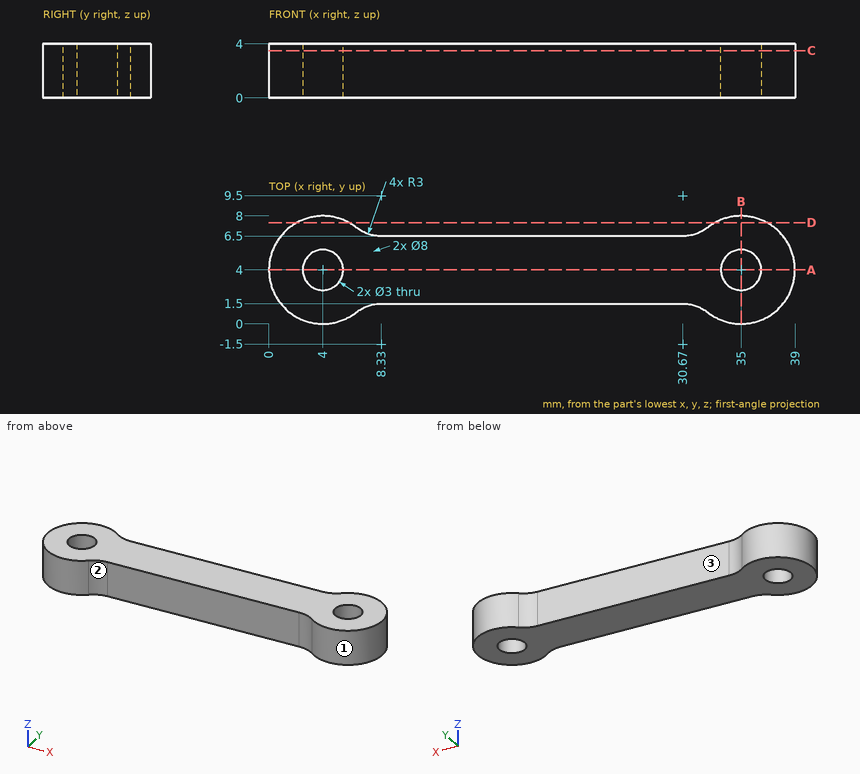
Check sheet for the drawn part. Datum: minimum x, y, z corner. Units: mm. A direction names the side the tool comes from. Round coordinates to 2 decimals unless told otherwise and drop trailing zeros. Loops run counter-clockwise (first coordinate to the right, second up) from the corner with the lowest first, then second, coordinate; pieces in that order, holes last. Notation, with made-up numbers: (-2.5, 43) - (15.5, 43) arc R32 ccw to (15.5, 82) - close; hole circle Ø11 at (17, 11.5). An arc over 180 degrees is marked (long way). Write each question's results on one line, items separated by ' | '. Start each with the question number.
Q1. Cross-section at B-B on x = 35. Enter the section's corners in (y, z), and give its area (3 significant figures).
Q2. Gauge pin test, flat ends, axial feed: P1, Ø1.5, axis at x = 21, z = 1.5, coming from the -Y side; P2, Ø2.5, axis at x = 4, y = 4, coming from the +Z side; P3, Ø2, axis at y = 2.5, z = 3, coming from the +X side; P4, Ø1.2, axis at x = 20.5, z = 1.5, coming from the +Y side. Record the tip position at first contact, or that the pin passes through.
Q3. Cross-section at C-C on z = 3.5. Enter the section's corners in (x, y).
Q4. Thickness scan on line 1 (Y direction, x = 35, z = 3.2); line 2 (X direction, y = 2.75, z = 2.75); line 3 (X direction, y = 3.5, z = 1.1). Record the ranges inside material, lowest first. Write a range as [from, to].
Q5. Cross-section at A-A on y = 4. Enter the section's corners in (x, z).
Q6. Cross-section at D-D on y = 7.5. Enter the section's corners in (x, z).
Q7. Access from +Z, -Z, +X, -X, +Y, -Y to the whole of each face (thin tool, end or side, straight path). Record for the marked faces 1, 2 and 3.
Answers below:
1) outline: (0, 0) - (2.5, 0) - (2.5, 4) - (0, 4) - close; (5.5, 0) - (8, 0) - (8, 4) - (5.5, 4) - close | area: 20.0 mm²
2) P1: stops at y = 1.5 | P2: passes through | P3: stops at x = 38.97 | P4: stops at y = 6.5
3) outline: (6.47, 0.86) arc R3 cw to (8.33, 1.5) - (30.67, 1.5) arc R3 cw to (32.53, 0.86) arc R4 ccw (long way) to (32.53, 7.14) arc R3 cw to (30.67, 6.5) - (8.33, 6.5) arc R3 cw to (6.47, 7.14) arc R4 ccw (long way) to start; hole circle Ø3 at (4, 4); hole circle Ø3 at (35, 4)
4) line 1: y = [0, 2.5], [5.5, 8] | line 2: x = [0.2, 3.17], [4.83, 34.17], [35.83, 38.8] | line 3: x = [0.03, 2.59], [5.41, 33.59], [36.41, 38.97]
5) outline: (0, 0) - (2.5, 0) - (2.5, 4) - (0, 4) - close; (5.5, 0) - (33.5, 0) - (33.5, 4) - (5.5, 4) - close; (36.5, 0) - (39, 0) - (39, 4) - (36.5, 4) - close
6) outline: (2.06, 0) - (5.94, 0) - (5.94, 4) - (2.06, 4) - close; (33.06, 0) - (36.94, 0) - (36.94, 4) - (33.06, 4) - close
7) face 1: +Z, -Z | face 2: +Z, -Z, -Y | face 3: +Z, -Z, +Y
